The model under review builds one solid part; all positions refer to its coordinate system, in mm. Face numbers are marked on the shaded views. A direction names the side the tool comes from. Round coordinates to 2 decimals unless told otherwise and drop trailing zeros. Order: outer loops, then holes, each group sorted by start corner. A loop starts at its lowest first (then second) coordinate and runs counter-clockwise, first axis right, second up. Notation, with made-up numbers: (9, 20) - (41, 20) arc R15 ccw to (41, 32) - close; hole circle Ø1 at (1.5, 85). An arc over 180 degrees is marked (long way). One line per question, with ' | ' between items. Start each with the question number.
Item 1: Add section D-D on x = -11. State the section outline as (y, z) points, and give its area (3 significant figures).
Item 2: Add section C-C on x = -22. State how many separate pieces and enclosed holes the cut face has, and give its area (3 significant figures).
Item 3: Tool access review of the marked faces 1, 2 and 3: name each direction out of +Z, -Z, +X, -X, +Y, -Y from which nothing blocks a thin tool from reaching the whole face with its end or side.
Item 4: For L1, parallel to Y at x = -30.5, z = 51; L2, parallel to Y at x = -32, z = 15; L3, parallel to Z at x = -8.5, y = -4, list the stretches that pass through material, from the lowest coordinate up. Write a range as [from, to].
Item 5: Insertion check: pin 1 Ø12 at (x, z) = (-30.5, 29) entering from -Y; pin 2 Ø6 at (x, z) = (-16, 53) entering from +Y; pin 3 Ø12.5 at (x, y) = (-21, 28.5) entering from +Z. Each pin has a flat end and moves straight along its axis. Give the tip position at first contact, or say it passes through.
Item 6: Add section B-B on z = 26. State the section outline as (x, y) points, and give its area (3 significant figures).
Item 7: Draft analysis for pull direction Y (two halves, no side actions). For the marked faces 4, 5, 6 and 7, state which applies: +Y half, -Y half, draft (parallel to the pull), parting line (faces both ways), or undercut.
Item 8: Add section A-A on z = 40. State the section outline as (x, y) points, and give its area (3 significant figures).
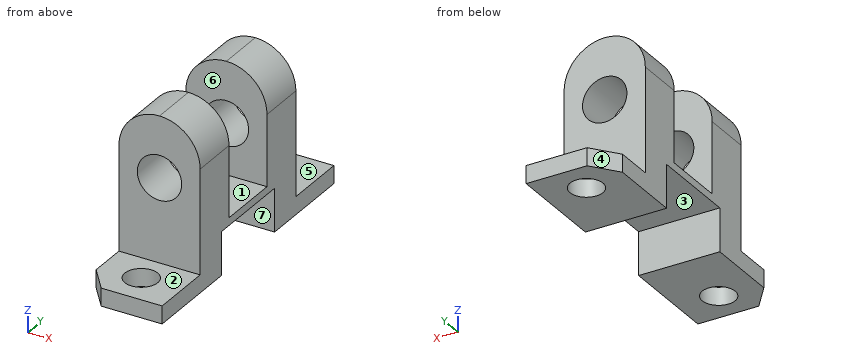
from build123d import *

# Parameters (mm, degrees)
F0_W      = 32
F0_H      = 113
F1_DEPTH  = 20
F2_W      = 32
F2_H      = 25
F3_DEPTH  = 13
F4_W      = 32
F4_H      = 35
F5_DEPTH  = 17
F6_W      = 32
F6_H      = 19
F7_DEPTH  = 44
F8_R      = 16
F9_R      = 15.99999
F10_R     = 16
F11_R     = 15.99999
F12_R     = 6.5
F13_DEPTH = 13
F14_R     = 6.5
F15_DEPTH = 13
F17_DEPTH = 25
F19_DEPTH = 25
F20_R     = 8.75
F21_DEPTH = 100


# Not quite as in the source:
# - a fillet or chamfer is up to 0.001 mm smaller than in the source, because OpenCascade refuses the exact size


with BuildPart() as f1:
    # F0 (on Top) → F1 (new body)
    with BuildSketch(Plane.XY):
        with Locations((-23.4775710851, 33.1401875504)):
            Rectangle(F0_W, F0_H)
    extrude(amount=F1_DEPTH)

    # F2 (on face) → F3 (cut)
    with BuildSketch(Plane.XY.offset(20)):
        with Locations((-23.4775710851, 77.1401875504)):
            Rectangle(F2_W, F2_H)
        with Locations((-23.4775710851, -10.8598124496)):
            Rectangle(F2_W, F2_H)
    extrude(amount=-F3_DEPTH, mode=Mode.SUBTRACT)

    # F4 (on face) → F5 (cut)
    with BuildSketch(Plane(origin=(0, 0, 0), x_dir=(1, 0, 0), z_dir=(0, 0, -1))):
        with Locations((-23.4775710851, -33.1401875504)):
            Rectangle(F4_W, F4_H)
    extrude(amount=-F5_DEPTH, mode=Mode.SUBTRACT)

    # F6 (on face) → F7 (join)
    with BuildSketch(Plane.XY.offset(20)):
        with Locations((-23.4775710851, 55.1401875504)):
            Rectangle(F6_W, F6_H)
        with Locations((-23.4775710851, 11.1401875504)):
            Rectangle(F6_W, F6_H)
    extrude(amount=F7_DEPTH)

    # F8
    f8_edges = [f1.edges().sort_by_distance(p)[0] for p in [
        (-39.477571, 55.140188, 64),
    ]]
    fillet(f8_edges, radius=F8_R)

    # F9 (radius 16 in the source; OpenCascade refuses exactly that, so slightly less here)
    f9_edges = [f1.edges().sort_by_distance(p)[0] for p in [
        (-7.477571, 55.140188, 64),
    ]]
    fillet(f9_edges, radius=F9_R)

    # F10
    f10_edges = [f1.edges().sort_by_distance(p)[0] for p in [
        (-39.477571, 11.140188, 64),
    ]]
    fillet(f10_edges, radius=F10_R)

    # F11 (radius 16 in the source; OpenCascade refuses exactly that, so slightly less here)
    f11_edges = [f1.edges().sort_by_distance(p)[0] for p in [
        (-7.477571, 11.140188, 64),
    ]]
    fillet(f11_edges, radius=F11_R)

    # F12 (on face) → F13 (cut)
    with BuildSketch(Plane.XY.offset(7)):
        with Locations((-23.4775710851, -10.3598124496)):
            Circle(F12_R)
    extrude(amount=-F13_DEPTH, mode=Mode.SUBTRACT)

    # F14 (on face) → F15 (cut)
    with BuildSketch(Plane.XY.offset(7)):
        with Locations((-23.4775710851, 76.6401875504)):
            Circle(F14_R)
    extrude(amount=-F15_DEPTH, mode=Mode.SUBTRACT)

    # F16 (on face) → F17 (cut)
    with BuildSketch(Plane.XY.offset(7)):
        Polygon((-39.4775710851, -13.3598124496), (-39.4775710851, -23.3598124496), (-31.4775710851, -23.3598124496), align=None)
    extrude(amount=-F17_DEPTH, mode=Mode.SUBTRACT)

    # F18 (on face) → F19 (cut)
    with BuildSketch(Plane.XY.offset(7)):
        Polygon((-31.4775710851, 89.6401875504), (-39.4775710851, 89.6401875504), (-39.4775710851, 79.6401875504), align=None)
    extrude(amount=-F19_DEPTH, mode=Mode.SUBTRACT)

    # F20 (on face) → F21 (cut)
    with BuildSketch(Plane.XZ.offset(-1.6401875504)):
        with Locations((-23.4775710851, 40)):
            Circle(F20_R)
    extrude(amount=-F21_DEPTH, mode=Mode.SUBTRACT)


solid = f1.part
Determined:
1) outline: (-23.36, 0) - (15.64, 0) - (15.64, 17) - (50.64, 17) - (50.64, 0) - (89.64, 0) - (89.64, 7) - (64.64, 7) - (64.64, 58.02) - (45.64, 58.02) - (45.64, 20) - (20.64, 20) - (20.64, 58.02) - (1.64, 58.02) - (1.64, 7) - (-23.36, 7) - close | area: 2,460 mm2
2) separate pieces: 5 | enclosed holes: 0 | area: 1,850 mm2
3) face 1: +Z, +X, -X | face 2: +Z, +X, -X, -Y | face 3: -Z, +X, -X
4) L1: [1.64, 20.64], [45.64, 64.64] | L2: [1.64, 15.64], [50.64, 64.64] | L3: [0, 7]
5) pin 1: y = 1.64 | pin 2: y = 64.64 | pin 3: z = 20
6) outline: (-39.48, 1.64) - (-7.48, 1.64) - (-7.48, 20.64) - (-39.48, 20.64) - close; (-39.48, 45.64) - (-7.48, 45.64) - (-7.48, 64.64) - (-39.48, 64.64) - close | area: 1,220 mm2
7) face 4: +Y half | face 5: draft | face 6: undercut | face 7: undercut
8) outline: (-39.48, 1.64) - (-32.23, 1.64) - (-32.23, 20.64) - (-39.48, 20.64) - close; (-39.48, 45.64) - (-32.23, 45.64) - (-32.23, 64.64) - (-39.48, 64.64) - close; (-14.73, 1.64) - (-7.48, 1.64) - (-7.48, 20.64) - (-14.73, 20.64) - close; (-14.73, 45.64) - (-7.48, 45.64) - (-7.48, 64.64) - (-14.73, 64.64) - close | area: 551 mm2
